Input: part model. Units: mm. Frame: model coordinates. A direction names the side the tool comes from. Coordinates: 2 decimals unless noted, no trailing zeros. Loops run counter-clockwise (first coordinate to the right, second up) from the corner with the lowest first, then second, coordinate; pieces in that order, holes last. Notation, with made-up numbers: M 57,43 L 104,43 A33 ccw 104,72 Z; hole C 5,82.5 d5. An arc over 180 degrees is marked long. Use a Markdown table: item, result. Add a question column.
1. Section D-D on x = 23. Output: boundary loops of the cut face in (y, z), then the cut area to 3 significant figures.
2. Line query: L1, parallel to X at y = 2.9, z = -9; L2, parallel to Z at x = 43.5, y = 1.65; L3, parallel to X at y = 0.55, z = -8. Output: solid intervals per line, ascending. Write a range as [from, to].
3. Set-up query: faces 4 (the flat face through (7, 3, -11)), 5 (the flat face through (7, 3, -1)), 6 (the cylindrical face through (3.57, 2.96, -4.6)). Return all of +Z, -Z, +X, -X, +Y, -Y with unobstructed straight access to the full face (end or side cutting, diameter ignored); none if empty.
4. Draft query along X for faces 1 (the flat face through (47, 3, -6)), 2 (the flat face through (3, 3, -12)), 3 (the flat face through (24, 3, -2.5)). Return one class per face: +X half, -X half, draft (parallel to the pull), parting line (faces both ways), or undercut.
5. Section A-A on x = 3.5. Output: boundary loops of the cut face in (y, z), then the cut area to 3 significant figures.
6. Section C-C on y = 3.4. Output: boundary loops of the cut face in (x, z), then the cut area to 3 significant figures.
7. Section B-B on z = -9. Output: boundary loops of the cut face in (x, y).
8. Pin query (flat end, axial travel): pin 1 (3 mm diameter, centred on x = 26.5, y = 3, fed in from +Z); pin 2 (3 mm diameter, centred on x = 43.5, z = -3, fed in from -Y). Return the tip coordinate at first contact, or that it passes through.
```python
from build123d import *

# Parameters (mm, degrees)
SKETCH1_R           = 1.6
BOSS_EXTRUDE1_DEPTH = 6
FILLET1_R           = 0.5


with BuildPart() as part:
    # Sketch1 → Boss-Extrude1 (new body)
    with BuildSketch(Plane(origin=(0, 0, 0), x_dir=(1, 0, 0), z_dir=(0, 1, 0))):
        Polygon((0, 0), (0, 12), (7, 12), (7, 9.5), (40, 9.5), (40, 12), (47, 12), (47, 0), (40, 0), (40, 2.5), (7, 2.5), (7, 0), align=None)
        with Locations(Location((3.5, 9, 0), (0, 0, 270))):
            Circle(SKETCH1_R, mode=Mode.SUBTRACT)
        with Locations(Location((3.5, 3, 0), (0, 0, 270))):
            Circle(SKETCH1_R, mode=Mode.SUBTRACT)
        with Locations(Location((43.5, 3, 0), (0, 0, 90))):
            Circle(SKETCH1_R, mode=Mode.SUBTRACT)
        with Locations(Location((43.5, 9, 0), (0, 0, 90))):
            Circle(SKETCH1_R, mode=Mode.SUBTRACT)
    extrude(amount=BOSS_EXTRUDE1_DEPTH)

    # Fillet1
    fillet1_edges = [part.edges().sort_by_distance(p)[0] for p in [
        (7, 3, -9.5),
        (40, 3, -9.5),
        (40, 3, -2.5),
        (7, 3, -2.5),
    ]]
    fillet(fillet1_edges, radius=FILLET1_R)


solid = part.part
```
Answers below:
| question | item | result |
|---|---|---|
| 1 | outline | M 0,-9.5 L 6,-9.5 L 6,-2.5 L 0,-2.5 Z |
| 1 | area | 42.0 mm² |
| 2 | L1 | x = [0, 1.9], [5.1, 41.9], [45.1, 47] |
| 2 | L2 | z = [-12, -10.6], [-7.4, -4.6], [-1.4, 0] |
| 2 | L3 | x = [0, 2.25], [4.75, 42.25], [44.75, 47] |
| 3 | face 4 | -Z, +Y, -Y |
| 3 | face 5 | +Z, +Y, -Y |
| 3 | face 6 | +Y, -Y |
| 4 | face 1 | +X half |
| 4 | face 2 | draft |
| 4 | face 3 | undercut |
| 5 | outline | M 0,-12 L 6,-12 L 6,-10.6 L 0,-10.6 Z; M 0,-7.4 L 6,-7.4 L 6,-4.6 L 0,-4.6 Z; M 0,-1.4 L 6,-1.4 L 6,0 L 0,0 Z |
| 5 | area | 33.6 mm² |
| 6 | outline | M 0,-12 L 7,-12 L 7,-10 A0.5 cw 7.5,-9.5 L 39.5,-9.5 A0.5 cw 40,-10 L 40,-12 L 47,-12 L 47,0 L 40,0 L 40,-2 A0.5 cw 39.5,-2.5 L 7.5,-2.5 A0.5 cw 7,-2 L 7,0 L 0,0 Z; hole C 3.5,-9 d3.2; hole C 3.5,-3 d3.2; hole C 43.5,-9 d3.2; hole C 43.5,-3 d3.2 |
| 6 | area | 367 mm² |
| 7 | outline | M 0,0 L 1.9,0 L 1.9,6 L 0,6 Z; M 5.1,0 L 41.9,0 L 41.9,6 L 5.1,6 Z; M 45.1,0 L 47,0 L 47,6 L 45.1,6 Z |
| 8 | pin 1 | stops at z = -2.5 |
| 8 | pin 2 | passes through |
